Verification items for the finished model (mm, model axes). A direction names the side the tool comes from. Coordinates: 2 decimals unless noted, no trailing zeros. Write each loop counter-clockwise with the first axis right and the second up, starting at its lowest first coordinate (ties: lowest second). Pieces come first, ordered by that corner, then holes.
```python
from build123d import *

# Parameters (mm, degrees)
SKETCH033_W     = 46
SKETCH033_H     = 41
PAD022_DEPTH    = 3
POCKET011_DEPTH = 5
PAD023_DEPTH    = 47
SKETCH036_W     = 46
SKETCH036_H     = 41
PAD024_DEPTH    = 3
SKETCH037_R     = 1.55
POCKET012_DEPTH = 5
POCKET013_DEPTH = 41.001
SKETCH039_W     = 22
SKETCH039_H     = 40
POCKET014_DEPTH = 5


with BuildPart() as part:
    # Sketch033 (on Face1 of Binder006) → Pad022 (new body)
    with BuildSketch(Plane(origin=(0, 0, 3.2), x_dir=(1, 0, 0), z_dir=(0, 0, -1))):
        with Locations((-83.6396103068, -83.6396103068)):
            Rectangle(SKETCH033_W, SKETCH033_H)
    extrude(amount=PAD022_DEPTH)

    # Sketch034 → Pocket011 (cut)
    with BuildSketch(Plane.XY):
        Polygon((-91.4177848998, 95.660425587), (-95.660425587, 91.4177848998), (-91.4177848998, 87.1751442127), (-87.1751442127, 91.4177848998), align=None)
        Polygon((-75.8614357137, 95.660425587), (-80.1040764009, 91.4177848998), (-75.8614357137, 87.1751442127), (-71.6187950266, 91.4177848998), align=None)
        Polygon((-91.4177848998, 80.1040764009), (-95.660425587, 75.8614357137), (-91.4177848998, 71.6187950266), (-87.1751442127, 75.8614357137), align=None)
        Polygon((-80.1040764009, 75.8614357137), (-75.8614357137, 71.6187950266), (-71.6187950266, 75.8614357137), (-75.8614357137, 80.1040764009), align=None)
    extrude(amount=POCKET011_DEPTH, mode=Mode.SUBTRACT)

    # Sketch035 (on Face5 of Pocket011) → Pad023 (join)
    with BuildSketch(Plane(origin=(0, 0, 0.2), x_dir=(1, 0, 0), z_dir=(0, 0, -1))):
        Polygon((-60.6396103068, -63.1396103068), (-106.6396103068, -63.1396103068), (-106.6396103068, -104.1396103068), (-60.6396103068, -104.1396103068), (-60.6396103068, -101.1396103068), (-103.6396103068, -101.1396103068), (-103.6396103068, -66.1396103068), (-60.6396103068, -66.1396103068), align=None)
    extrude(amount=PAD023_DEPTH)

    # Sketch036 (on Face20 of Pad023) → Pad024 (join)
    with BuildSketch(Plane(origin=(0, 0, -46.8), x_dir=(1, 0, 0), z_dir=(0, 0, -1))):
        with Locations((-83.63961, -83.63961)):
            Rectangle(SKETCH036_W, SKETCH036_H)
    extrude(amount=-PAD024_DEPTH)

    # Sketch037 (on Face27 of Pad024) → Pocket012 (cut)
    with BuildSketch(Plane(origin=(0, 0, -46.8), x_dir=(1, 0, 0), z_dir=(0, 0, -1))):
        with Locations((-98.8896103068, -71.6396103068)):
            Circle(SKETCH037_R)
        with Locations((-68.3896103068, -71.6396103068)):
            Circle(SKETCH037_R)
        with Locations((-98.8896103068, -95.6396103068)):
            Circle(SKETCH037_R)
        with Locations((-68.3896103068, -95.6396103068)):
            Circle(SKETCH037_R)
    extrude(amount=-POCKET012_DEPTH, mode=Mode.SUBTRACT)

    # Sketch038 (on Face27 of Pocket012) → Pocket013 (cut, through all)
    with BuildSketch(Plane(origin=(0, 104.1396103068, 0), x_dir=(-1, 0, 0), z_dir=(0, 1, 0))):
        Polygon((81.6396103068, 0.2), (59.6396103068, 0.2), (59.6396103068, -43.8), (81.6396103068, -43.8), (96.6396103068, -28.8), (96.6396103068, -14.8), align=None)
    extrude(amount=-POCKET013_DEPTH, mode=Mode.SUBTRACT)

    # Sketch039 (on Face30 of Pocket013) → Pocket014 (cut)
    with BuildSketch(Plane(origin=(-106.6396103068, 0, 0), x_dir=(0, -1, 0), z_dir=(-1, 0, 0))):
        with Locations((-83.6396103068, -21.8)):
            Rectangle(SKETCH039_W, SKETCH039_H)
    extrude(amount=-POCKET014_DEPTH, mode=Mode.SUBTRACT)


solid = part.part
```
1. Sectioned sample at A-A, the plane z = -27. Record the boundary of the cut face in (x, y).
2. Draft check along X on faces 1 (the flat face through (-96.64, 65, -22)), 2 (the flat face through (-82, 84, -43.8)), 3 (the flat face through (-89.326, 89.267, 1.679)). Enter one of: pulls with the +X half, pulls with the -X half, needs draft (parallel to the pull), parting line crosses it, or undercut.
3. Sectioned sample at D-D, the plane y = 77. Record the boundary of the cut face in (x, z).
4. Sectioned sample at C-C, the plane x = -64.5. Record the boundary of the cut face in (y, z).
5. Material ranges on L1, parallel to Y at x = -87, z = -39; L2, parallel to Z at x = -62.5, y = 88.5; L3, parallel to X at y = 102.5, z = -16.5, recorded low to high.
6. Sectioned sample at B-B, the plane y = 83. Record the boundary of the cut face in (x, z).
7. Gauge pin test, flat ends, axial feed: P1, Ø0.9, axis at y = 65, z = -19.5, coming from the +X side; P2, Ø1.9, axis at x = -98.89, y = 95.64, coming from the -Z side. Record the tip position at first contact, or that the pin passes through.
8. Tool access check on faces 4 (the cylindrical face through (-99.091, 70.103, -45.321)), 5 (the flat face through (-89.326, 73.71, 1.679)), 6 (the flat face through (-89.035, 102.661, -36.405)). Record the directions out of +Z, -Z, +X, -X, +Y, -Y that give a thin tool (end or side, any length) a straight path to the whole face; none if there is none.
Outcome:
1. outline: (-106.64, 63.14) - (-96.64, 63.14) - (-96.64, 66.14) - (-103.64, 66.14) - (-103.64, 72.64) - (-106.64, 72.64) - close; (-106.64, 94.64) - (-103.64, 94.64) - (-103.64, 101.14) - (-96.64, 101.14) - (-96.64, 104.14) - (-106.64, 104.14) - close
2. face 1: pulls with the +X half
2. face 2: needs draft
2. face 3: undercut
3. outline: (-106.64, -46.8) - (-60.64, -46.8) - (-60.64, -43.8) - (-103.64, -43.8) - (-103.64, -41.8) - (-106.64, -41.8) - close; (-106.64, -1.8) - (-103.64, -1.8) - (-103.64, 0.2) - (-94.52, 0.2) - (-94.52, 3.2) - (-106.64, 3.2) - close; (-88.31, 0.2) - (-78.97, 0.2) - (-78.97, 3.2) - (-88.31, 3.2) - close; (-72.76, 0.2) - (-60.64, 0.2) - (-60.64, 3.2) - (-72.76, 3.2) - close
4. outline: (63.14, -46.8) - (104.14, -46.8) - (104.14, -43.8) - (63.14, -43.8) - close; (63.14, 0.2) - (104.14, 0.2) - (104.14, 3.2) - (63.14, 3.2) - close
5. L1: y = 63.14 to 66.14, 101.14 to 104.14
5. L2: z = -46.8 to -43.8, 0.2 to 3.2
5. L3: x = -106.64 to -96.64
6. outline: (-106.64, -46.8) - (-60.64, -46.8) - (-60.64, -43.8) - (-103.64, -43.8) - (-103.64, -41.8) - (-106.64, -41.8) - close; (-106.64, -1.8) - (-103.64, -1.8) - (-103.64, 0.2) - (-60.64, 0.2) - (-60.64, 3.2) - (-106.64, 3.2) - close
7. P1: stops at x = -96.64
7. P2: stops at z = 0.2
8. face 4: -Z
8. face 5: +Z
8. face 6: +X, +Y, -Y
